Build history of the part. All positions in model axes, mm. A direction names the side the tool comes from. Give positions to 0.01 mm unless a question says otherwise; leave off trailing zeros. Order: outer loops, then holes, each group sorted by start corner. A loop starts at its lowest first (then second) coordinate and runs counter-clockwise, first axis right, second up. Notation, with made-up numbers: (26, 35.5) - (66, 35.5) arc R16 cw to (66, 56.5) - close; hole circle Ø4 at (78, 89). An arc over 180 degrees is marked (long way). Use a Markdown table: item, result.
Autodesk Inventor part; units mm, degrees
ref_plane "YZ Plane" through (0, 0, 0) normal (1, 0, 0) x (0, 1, 0)
ref_plane "XZ Plane" through (0, 0, 0) normal (0, 1, 0) x (-1, 0, 0)
ref_plane "XY Plane" through (0, 0, 0) normal (0, 0, 1) x (1, 0, 0)
sketch "Sketch1" plane through (0, 0, 0) normal (0, 0, 1) x (1, 0, 0)
  line L0 (-5, 0) -> (5, 0) construction
  line L1 (-5, -1) -> (5, -1)
  line L2 (5, 1) -> (-5, 1)
  arc A0 (-5, 1) -> (-5, -1) centre (-5, 0) ccw
  arc A1 (5, -1) -> (5, 1) centre (5, 0) ccw
  line L3 (-5, 0) -> (5, 0) construction
  line L4 (-5, -2) -> (5, -2)
  line L5 (5, 2) -> (-5, 2)
  arc A2 (-5, 2) -> (-5, -2) centre (-5, 0) ccw
  arc A3 (5, -2) -> (5, 2) centre (5, 0) ccw
  point P0 (0, 0)
extrude "Extrusion1" add sketch "Sketch1" along normal blind 2 contours A0 L2 A1 L1 | A2 L5 A3 L4
sketch "Sketch2" plane through (0, 0, 0) normal (0, 0, -1) x (-1, 0, 0)
  arc A0 (5, -2) -> (5, 2) centre (5, 0) ccw
  line L0 (-5, 0) -> (5, 0) construction
  line L1 (-5, -1) -> (5, -1)
  line L2 (5, 1) -> (-5, 1)
  arc A1 (-5, 1) -> (-5, -1) centre (-5, 0) ccw
  arc A2 (5, -1) -> (5, 1) centre (5, 0) ccw
  line L3 (5, 1) -> (5, -1)
  line L4 (-5, -1) -> (-5, 1)
  point P0 (0, 0)
extrude "Extrusion2" add sketch "Sketch2" along normal blind 10 contours L4 L2 L3 L1
sketch "Sketch3" plane through (5, -1, 0) normal (1, 0, 0) x (0, 0, -1)
  line L0 (0, 2) -> (10, 2)
  line L1 (10, 2) -> (8.5, 2)
  line L2 (8.5, 2) -> (8.5, 2.5)
  line L3 (8.5, 2.5) -> (10, 2)
  line L4 (0, 0) -> (10, 0)
  line L5 (10, 0) -> (8.5, 0)
  line L6 (8.5, 0) -> (8.5, -0.5)
  line L7 (8.5, -0.5) -> (10, 0)
  point P0 (0, 1)
  dimension "d8" = 1.5
  dimension "d9" = 0.5
  dimension "d10" = 0.5
extrude "Extrusion3" add sketch "Sketch3" against normal up to surface (10 mm away)
sketch "Sketch4" plane through (5, -1, 0) normal (1, 0, 0) x (0, 0, -1)
  line L0 (10, 0) -> (10, 2)
  line L1 (10, 1) -> (10, 1.5)
  line L2 (10, 1.5) -> (0, 1)
  line L3 (10, 1) -> (10, 0.5)
  line L4 (10, 0.5) -> (0, 1)
  dimension "d13" = 0.5
  dimension "d14" = 0.5
extrude "Extrusion4" cut sketch "Sketch4" against normal through all
properties part number "clip"
1) Pin check, flat tips, straight feed: P1, Ø1.2, axis at y = 1, z = -5.5, coming from the -X side; P2, Ø2.5, axis at x = 1, z = -2.5, coming from the +Y side; P3, Ø0.8, axis at y = -1, z = -2.5, coming from the +X side. Stop position of each tip, or through.
Computed:
| item | result |
|---|---|
| P1 | stops at x = -5 |
| P2 | stops at y = 1 |
| P3 | stops at x = 5 |
2) Slice it at C-C (y = -1.3). Write the cut outline in (x, z), and give its area (3 significant figures).
Computed:
| item | result |
|---|---|
| outline | (-6.52, 0) - (6.52, 0) - (6.52, 2) - (-6.52, 2) - close; (-5, -9.1) - (5, -9.1) - (5, -8.5) - (-5, -8.5) - close |
| area | 32.1 mm² |
3) Wall check: line 1 (X direction, y = 0.25, z = -1); line 2 (Y direction, x = 0.25, z = -8.25); line 3 (Y direction, x = 3.5, z = -5). Give the ranges that are in metal, low to high. Write a range as from..to.
Computed:
| item | result |
|---|---|
| line 1 | x = -5..5 |
| line 2 | y = -1..-0.41, 0.41..1 |
| line 3 | y = -1..-0.25, 0.25..1 |
4) Slice it at A-A (z = -7). Write the cut outline in (x, y).
Computed:
| item | result |
|---|---|
| outline | (-5, -1) - (5, -1) - (5, -0.35) - (-5, -0.35) - close; (-5, 0.35) - (5, 0.35) - (5, 1) - (-5, 1) - close |
5) Two-plate mould, pull along Z, no slides. Class faces 1 (the flat face through (0, -2, 1)), 2 (the flat face through (-0.1, 1.4, 0)), 3 (the flat face through (0, 0, 2)): +Z half, -Z half, draft (parallel to the pull), parting line (faces both ways), or undercut.
Computed:
| item | result |
|---|---|
| face 1 | draft |
| face 2 | undercut |
| face 3 | +Z half |
6) Tool access for faces 4 (the flat face through (-5, -0.6, -4.9)), 5 (the flat face through (5, 0.6, -4.9)), 6 (the flat face through (0, 1, -4)), 7 (the flat face through (0.07, 1.253, -9.24)), 8 (the flat face through (0, -1, -4)): list every direction of +Z, -Z, +X, -X, +Y, -Y with a clear straight run to the whole face (end or side of a thin tool).
Computed:
| item | result |
|---|---|
| face 4 | -Z, -X, +Y, -Y |
| face 5 | -Z, +X, +Y, -Y |
| face 6 | +X, -X, +Y |
| face 7 | -Z, +X, -X, +Y |
| face 8 | +X, -X, -Y |
7) Slice it at B-B (x = 0.75). Write the cut outline in (y, z), and give its area (4 significant figures).
Computed:
| item | result |
|---|---|
| outline | (-2, 0) - (-1, 0) - (-1, -8.5) - (-1.5, -8.5) - (-1, -10) - (-0.5, -10) - (0, 0) - (0.5, -10) - (1, -10) - (1.5, -8.5) - (1, -8.5) - (1, 0) - (2, 0) - (2, 2) - (-2, 2) - close |
| area | 23.75 mm² |
